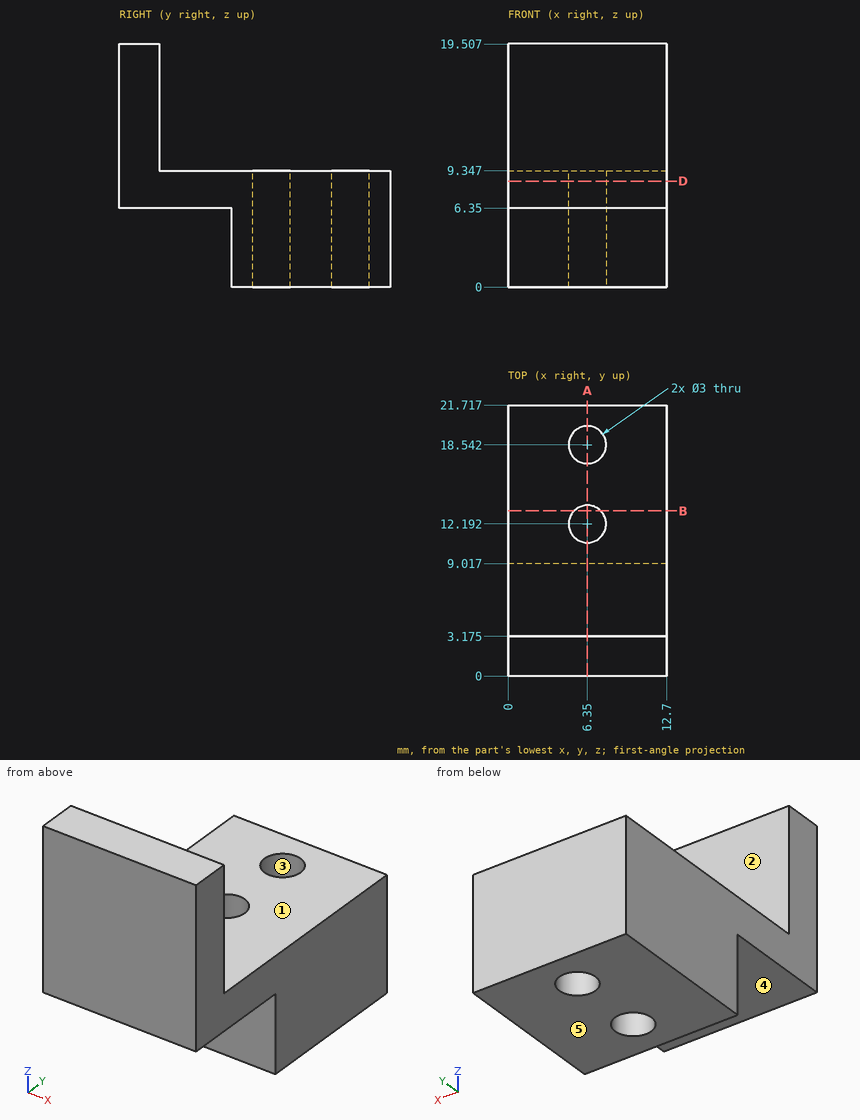
Geometry check sheet. Reference: drawing and pictorial views, mm from the part's lowest x, y, z. A direction names the side the tool comes from. Round coordinates to 2 decimals unless told otherwise and drop trailing zeros. Order: outer loops, then holes, each group sorted by start corner. A loop starts at its lowest first (then second) coordinate and runs counter-clockwise, first axis right, second up. Notation, with made-up numbers: M 26.25,36.5 L 64.25,36.5 A26 ccw 64.25,65.5 Z; hole C 66,56 d9. An arc over 180 degrees is marked long. Answer as CSV lines item,"result".
1) Sectioned sample at D-D on z = 8.5. Record the cut outline in (x, y).
Entries:
outline,"M 0,0 L 12.7,0 L 12.7,21.72 L 0,21.72 Z; hole C 6.35,12.19 d3; hole C 6.35,18.54 d3"
2) Mould release check, pull along Y, two halves, no side actions. Record for the marked faces 1, 2 and 3: +Y half, -Y half, draft (parallel to the pull), parting line (faces both ways), or undercut.
Entries:
face 1,"draft"
face 2,"+Y half"
face 3,"undercut"
3) Tool access check on the marked faces 4 and 5. Record the directions out of +Z, -Z, +X, -X, +Y, -Y that give a thin tool (end or side, any length) a straight path to the whole face; none if there is none.
Entries:
face 4,"-Z, +X, -X, -Y"
face 5,"-Z, +X, -X, +Y, -Y"
4) Thickness scan on probe 1 along Y at (x, z) = (6.35, 6.5); probe 2 along Y at (x, z) = (6.35, 6.25); probe 3 along Y at (x, z) = (8.5, 1.75). Record the ranges inside material, lowest first. Write a range as [from, to].
Entries:
probe 1,"[0, 10.69], [13.69, 17.04], [20.04, 21.72]"
probe 2,"[9.02, 10.69], [13.69, 17.04], [20.04, 21.72]"
probe 3,"[9.02, 21.72]"
5) Sectioned sample at B-B on y = 13.25. Record the cut outline in (x, z).
Entries:
outline,"M 0,0 L 5.29,0 L 5.29,9.35 L 0,9.35 Z; M 7.41,0 L 12.7,0 L 12.7,9.35 L 7.41,9.35 Z"
6) Sectioned sample at A-A on x = 6.35. Give the number of separate pieces and of enclosed holes in the cut face, and give its area (3 significant figures).
Entries:
separate pieces,"3"
enclosed holes,"0"
area,"122 mm2"
7) Gauge pin test, flat ends, axial feed: pin 1 Ø2.5 at (x, y) = (6.5, 4.5) entering from -Z; pin 2 Ø5 at (x, y) = (6.35, 12.192) entering from +Z; pin 3 Ø7 at (x, z) = (6.5, 2) entering from -Y. Record the tip position at first contact, or that the pin passes through.
Entries:
pin 1,"z = 6.35"
pin 2,"z = 9.35"
pin 3,"y = 9.02"
